Model file for the job. Use its own axes, mm. A direction names the side the tool comes from. Round coordinates to 2 decimals unless told otherwise and drop trailing zeros. Order: outer loops, then holes, each group sorted by start corner. A loop starts at its lowest first (then second) coordinate and runs counter-clockwise, first axis right, second up. Notation, with made-up numbers: (89.5, -17.5) - (129.5, -17.5) arc R16 ccw to (129.5, -12.5) - close; hole circle Ø11 at (-21.5, 37). An arc over 180 degrees is marked (long way). Write item = value, one per line. Start each with the question number.
from build123d import *

# Parameters (mm, degrees)
BOSS_EXTRUDE2_DEPTH = 4
BOSS_EXTRUDE3_START = 25
BOSS_EXTRUDE3_DEPTH = 25
BOSS_EXTRUDE4_START = 25
BASE_SKETCH_4_R     = 50
BASE_SKETCH_4_R_2   = 40
BASE_SKETCH_4_R_3   = 10
BOSS_EXTRUDE4_DEPTH = 40
BOSS_EXTRUDE5_START = 65
BASE_SKETCH_5_R     = 50
BASE_SKETCH_5_R_2   = 40
BASE_SKETCH_5_R_3   = 10
BOSS_EXTRUDE5_DEPTH = 5
BOSS_EXTRUDE6_START = 70
BASE_SKETCH_7_R     = 50
BASE_SKETCH_7_R_2   = 40
BOSS_EXTRUDE6_DEPTH = 100
FILLET1_R           = 10
FILLET2_R           = 10


with BuildPart() as part:
    # Base_Sketch → Boss-Extrude2 (new body)
    with BuildSketch(Plane.XY):
        with BuildLine():
            Line((34.641016151, 80), (17.320508076, 110))
            Line((17.320508076, 110), (-17.320508076, 110))
            Line((-17.320508076, 110), (-34.641016151, 80))
            ThreePointArc((-34.641016151, 80), (-41.961524227, 72.679491924), (-51.961524227, 70))
            Line((-51.961524227, 70), (-86.602540378, 70))
            Line((-86.602540378, 70), (-103.923048454, 40))
            Line((-103.923048454, 40), (-86.602540378, 10))
            ThreePointArc((-86.602540378, 10), (-83.923048454, 0), (-86.602540378, -10))
            Line((-86.602540378, -10), (-103.923048454, -40))
            Line((-103.923048454, -40), (-86.602540378, -70))
            Line((-86.602540378, -70), (-51.961524227, -70))
            ThreePointArc((-51.961524227, -70), (-41.961524227, -72.679491924), (-34.641016151, -80))
            Line((-34.641016151, -80), (-17.320508076, -110))
            Line((-17.320508076, -110), (17.320508076, -110))
            Line((17.320508076, -110), (34.641016151, -80))
            ThreePointArc((34.641016151, -80), (41.961524227, -72.679491924), (51.961524227, -70))
            Line((51.961524227, -70), (86.602540378, -70))
            Line((86.602540378, -70), (103.923048454, -40))
            Line((103.923048454, -40), (86.602540378, -10))
            ThreePointArc((86.602540378, -10), (83.923048454, 0), (86.602540378, 10))
            Line((86.602540378, 10), (103.923048454, 40))
            Line((103.923048454, 40), (86.602540378, 70))
            Line((86.602540378, 70), (51.961524227, 70))
            ThreePointArc((51.961524227, 70), (41.961524227, 72.679491924), (34.641016151, 80))
        make_face()
    extrude(amount=-BOSS_EXTRUDE2_DEPTH)

    # Base_Sketch<3> → Boss-Extrude3 (add)
    with BuildSketch(Plane.XY.offset(BOSS_EXTRUDE3_START)):
        with BuildLine():
            Line((86.602540378, 10), (103.923048454, 40))
            Line((103.923048454, 40), (86.602540378, 70))
            Line((86.602540378, 70), (51.961524227, 70))
            ThreePointArc((51.961524227, 70), (41.961524227, 72.679491924), (34.641016151, 80))
            Line((34.641016151, 80), (17.320508076, 110))
            Line((17.320508076, 110), (-17.320508076, 110))
            Line((-17.320508076, 110), (-34.641016151, 80))
            ThreePointArc((-34.641016151, 80), (-41.961524227, 72.679491924), (-51.961524227, 70))
            Line((-51.961524227, 70), (-86.602540378, 70))
            Line((-86.602540378, 70), (-103.923048454, 40))
            Line((-103.923048454, 40), (-86.602540378, 10))
            ThreePointArc((-86.602540378, 10), (-83.923048454, 0), (-86.602540378, -10))
            Line((-86.602540378, -10), (-103.923048454, -40))
            Line((-103.923048454, -40), (-86.602540378, -70))
            Line((-86.602540378, -70), (-51.961524227, -70))
            ThreePointArc((-51.961524227, -70), (-41.961524227, -72.679491924), (-34.641016151, -80))
            Line((-34.641016151, -80), (-17.320508076, -110))
            Line((-17.320508076, -110), (17.320508076, -110))
            Line((17.320508076, -110), (34.641016151, -80))
            ThreePointArc((34.641016151, -80), (41.961524227, -72.679491924), (51.961524227, -70))
            Line((51.961524227, -70), (86.602540378, -70))
            Line((86.602540378, -70), (103.923048454, -40))
            Line((103.923048454, -40), (86.602540378, -10))
            ThreePointArc((86.602540378, -10), (83.923048454, 0), (86.602540378, 10))
        make_face()
        Polygon((-31.176914536, 80), (-15.588457268, 107), (15.588457268, 107), (31.176914536, 80), (15.588457268, 53), (-15.588457268, 53), align=None, mode=Mode.SUBTRACT)
        Polygon((53.693575035, 67), (84.870489571, 67), (100.458946839, 40), (84.870489571, 13), (53.693575035, 13), (38.105117767, 40), align=None, mode=Mode.SUBTRACT)
        Polygon((-84.870489571, 67), (-53.693575035, 67), (-38.105117767, 40), (-53.693575035, 13), (-84.870489571, 13), (-100.458946839, 40), align=None, mode=Mode.SUBTRACT)
        Polygon((-100.458946839, -40), (-84.870489571, -13), (-53.693575035, -13), (-38.105117767, -40), (-53.693575035, -67), (-84.870489571, -67), align=None, mode=Mode.SUBTRACT)
        Polygon((84.870489571, -13), (100.458946839, -40), (84.870489571, -67), (53.693575035, -67), (38.105117767, -40), (53.693575035, -13), align=None, mode=Mode.SUBTRACT)
        Polygon((-15.588457268, -107), (-31.176914536, -80), (-15.588457268, -53), (15.588457268, -53), (31.176914536, -80), (15.588457268, -107), align=None, mode=Mode.SUBTRACT)
    extrude(amount=-BOSS_EXTRUDE3_DEPTH)

    # Base_Sketch<4> → Boss-Extrude4 (add)
    # profile 1 of 3: a face of its own
    with BuildSketch(Plane.XY.offset(BOSS_EXTRUDE4_START)):
        Circle(BASE_SKETCH_4_R)
        Circle(BASE_SKETCH_4_R_2, mode=Mode.SUBTRACT)
    # profile 2 of 3: a face of its own
    with BuildSketch(Plane.XY.offset(BOSS_EXTRUDE4_START)):
        Circle(BASE_SKETCH_4_R_2)
        Circle(BASE_SKETCH_4_R_3, mode=Mode.SUBTRACT)
    # profile 3 of 3: a face of its own
    with BuildSketch(Plane.XY.offset(BOSS_EXTRUDE4_START)):
        Circle(BASE_SKETCH_4_R_3)
    extrude(amount=BOSS_EXTRUDE4_DEPTH)

    # Base_Sketch<5> → Boss-Extrude5 (add)
    # profile 1 of 3: a face of its own
    with BuildSketch(Plane.XY.offset(BOSS_EXTRUDE5_START)):
        Circle(BASE_SKETCH_5_R)
        Circle(BASE_SKETCH_5_R_2, mode=Mode.SUBTRACT)
    # profile 2 of 3: a face of its own
    with BuildSketch(Plane.XY.offset(BOSS_EXTRUDE5_START)):
        Circle(BASE_SKETCH_5_R_2)
        Circle(BASE_SKETCH_5_R_3, mode=Mode.SUBTRACT)
    # profile 3 of 3: a face of its own
    with BuildSketch(Plane.XY.offset(BOSS_EXTRUDE5_START)):
        Circle(BASE_SKETCH_5_R_3)
    extrude(amount=BOSS_EXTRUDE5_DEPTH)

    # Base_Sketch<7> → Boss-Extrude6 (add)
    with BuildSketch(Plane.XY.offset(BOSS_EXTRUDE6_START)):
        Circle(BASE_SKETCH_7_R)
        Circle(BASE_SKETCH_7_R_2, mode=Mode.SUBTRACT)
    extrude(amount=BOSS_EXTRUDE6_DEPTH)

    # Fillet1
    fillet1_edges = [part.edges().sort_by_distance(p)[0] for p in [
        (-15.588457268, 107, 12.5),
        (-31.176914536, 80, 12.5),
        (-15.588457268, 53, 12.5),
        (15.588457268, 53, 12.5),
        (31.176914536, 80, 12.5),
        (15.588457268, 107, 12.5),
        (-17.320508076, 110, 10.5),
        (17.320508076, 110, 10.5),
    ]]
    fillet(fillet1_edges, radius=FILLET1_R)

    # Fillet2
    fillet2_edges = [part.edges().sort_by_distance(p)[0] for p in [
        (-15.588457268, -107, 12.5),
        (15.588457268, -107, 12.5),
        (31.176914536, -80, 12.5),
        (15.588457268, -53, 12.5),
        (-15.588457268, -53, 12.5),
        (-31.176914536, -80, 12.5),
        (-100.458946839, -40, 12.5),
        (-84.870489571, -67, 12.5),
        (-53.693575035, -67, 12.5),
        (-38.105117767, -40, 12.5),
        (-53.693575035, -13, 12.5),
        (-84.870489571, -13, 12.5),
        (-84.870489571, 67, 12.5),
        (-100.458946839, 40, 12.5),
        (-84.870489571, 13, 12.5),
        (-53.693575035, 13, 12.5),
        (-38.105117767, 40, 12.5),
        (-53.693575035, 67, 12.5),
        (100.458946839, 40, 12.5),
        (84.870489571, 67, 12.5),
        (53.693575035, 67, 12.5),
        (38.105117767, 40, 12.5),
        (53.693575035, 13, 12.5),
        (84.870489571, 13, 12.5),
        (84.870489571, -13, 12.5),
        (53.693575035, -13, 12.5),
        (38.105117767, -40, 12.5),
        (53.693575035, -67, 12.5),
        (84.870489571, -67, 12.5),
        (100.458946839, -40, 12.5),
        (103.923048454, -40, 10.5),
        (86.602540378, -70, 10.5),
        (17.320508076, -110, 10.5),
        (-17.320508076, -110, 10.5),
        (-86.602540378, -70, 10.5),
        (-103.923048454, -40, 10.5),
        (-103.923048454, 40, 10.5),
        (-86.602540378, 70, 10.5),
        (86.602540378, 70, 10.5),
        (103.923048454, 40, 10.5),
    ]]
    fillet(fillet2_edges, radius=FILLET2_R)


solid = part.part
Item 1: Drop flat-ended pins along their axis: pin 1 (15.5 mm diameter, centred on x = -67.5, z = 13, fed in from -Y); pin 2 (12 mm diameter, centred on x = 48.5, y = -14, fed in from +Z); pin 3 (16 mm diameter, centred on x = -78.5, y = -29, fed in from +Z); pin 4 (8 mm diameter, centred on x = 4.5, y = -13, fed in from +Z). Give the stop position or say it passes through.
Item 2: Saw through at D-D, the plane x = -76. Give the cut face in (y, z), then the cut area to 3 significant figures.
Item 3: Which spindle directions (+Z, -Z, +X, -X, +Y, -Y) get a long thin tool onto all of the face, cutting with end or side? Do faces 4 (the face through (-45.97, -26.38, 12.68)), 5 (the face through (-27.323, 92.675, 10.703)). Say none if no direction does.
Item 4: Probe L1, parallel to Y at x = -64, z = 5; L2, parallel to Y at x = 0, z = 119.5; L3, parallel to Y at x = 92, z = 15.5. List the from-to ranges inside material, lowest first.
Item 5: Mould opens along Y. For faces 1 (the face through (29.63, -80.07, 12.32)), 2 (the face through (-66, 70, 11)), 3 (the face through (27.323, -92.675, 10.703)) say: +Y half, -Y half, draft (parallel to the pull), parting line (faces both ways), or undercut.
Item 6: Saw through at A-A, the plane y = 0. Give the cut face in (x, z).
Item 7: Saw through at C-C, the plane z = 73. Give the cut face in (x, y).
Item 8: Saw through at B-B, the plane x = 0. Give the cut face in (y, z), then the cut area to 3 significant figures.
Check sheet entries:
q1.pin_1 = -70
q1.pin_2 = 170
q1.pin_3 = 0
q1.pin_4 = 70
q2.outline = (-70, -4) - (70, -4) - (70, 25) - (67, 25) - (67, 0) - (13, 0) - (13, 25) - (-13, 25) - (-13, 0) - (-67, 0) - (-67, 25) - (-70, 25) - close
q2.area = 1,360 mm2
q3.face_4 = +Z
q3.face_5 = +Z, -Z, -X, +Y
q4.L1 = -70 to -67, -13 to 13, 67 to 70
q4.L2 = -50 to -40, 40 to 50
q4.L3 = -60.65 to -54.65, -25.35 to -19.35, 19.35 to 25.35, 54.65 to 60.65
q5.face_1 = undercut
q5.face_2 = +Y half
q5.face_3 = -Y half
q6.outline = (-83.92, -4) - (83.92, -4) - (83.92, 25) - (50, 25) - (50, 170) - (40, 170) - (40, 70) - (-40, 70) - (-40, 170) - (-50, 170) - (-50, 25) - (-83.92, 25) - close
q7.outline = circle Ø100 at (0, 0); hole circle Ø80 at (0, 0)
q8.outline = (-110, -4) - (110, -4) - (110, 25) - (107, 25) - (107, 0) - (53, 0) - (53, 25) - (50, 25) - (50, 170) - (40, 170) - (40, 70) - (-40, 70) - (-40, 170) - (-50, 170) - (-50, 25) - (-53, 25) - (-53, 0) - (-107, 0) - (-107, 25) - (-110, 25) - close
q8.area = 10,200 mm2
